Design review of the part built by this model. Coordinates are the model's own, in mm. Coordinates: 2 decimals unless noted, no trailing zeros. Write each loop counter-clockwise with the first axis right and the second up, starting at its lowest first coordinate (ties: lowest second). Pieces come first, ordered by that corner, then holes.
Q1. Take a section at B-B, the plane z = 11.5. Write out the cut boundary in (x, y), plus the area to 3 significant figures.
Q2. For L1, parallel to Y at x = 273.5, z = 12; L2, parallel to X at y = 145.5, z = 2.5; L3, parallel to X at y = 155, z = 15.5, list the stretches that pass through material, from the lowest coordinate up.
Q3. Take a section at A-A, the plane y = 76. Write out the cut boundary in (x, z), plus the area to 3 significant figures.
Q4. The part is to be moulded in two halves that separate along X. For faces 1 (the flat face through (804, 13, 3)), 2 (the flat face through (796, 11, 0)), say which applies: released by +X, released by -X, zero draft, split by the parting line, or undercut.
Q5. For pin 1 Ø12.5 at (x, z) = (1153.5, 11) entering from +Y; pin 2 Ø6.5 at (x, y) = (1587, 615.5) entering from +Z, all flat-tipped, find the tip position at first contact; note any pin that passes through.
Q6. Take a section at C-C, the plane x = 1246.5. Write out the cut boundary in (y, z), plus the area to 3 significant figures.
from build123d import *

# Parameters (mm, degrees)
F1_DEPTH = 1600
F3_DEPTH = 650
F5_DEPTH = 1600
F7_DEPTH = 650


with BuildPart() as f1:
    # F0 (on Right) → F1 (new body)
    with BuildSketch(Plane.YZ):
        Polygon((0, 25), (0, 0), (25, 0), (25, 3), (3, 3), (3, 25), align=None)
    extrude(amount=F1_DEPTH)

    # F2 (on Front) → F3 (join)
    with BuildSketch(Plane.XZ):
        Polygon((0, 25), (0, 0), (25, 0), (25, 3), (3, 3), (3, 25), align=None)
    extrude(amount=-F3_DEPTH)

    # F4 (on Right) → F5 (join)
    with BuildSketch(Plane.YZ):
        Polygon((600, 0), (600, 25), (597, 25), (597, 3), (575, 3), (575, 0), align=None)
    extrude(amount=F5_DEPTH)

    # F6 (on Front) → F7 (join)
    with BuildSketch(Plane.XZ):
        Polygon((1600, 0), (1600, 25), (1597, 25), (1597, 3), (1575, 3), (1575, 0), align=None)
    extrude(amount=-F7_DEPTH)


solid = f1.part
Responses:
1. outline: (0, 0) - (1600, 0) - (1600, 650) - (1597, 650) - (1597, 600) - (3, 600) - (3, 650) - (0, 650) - close; hole (3, 3) - (1597, 3) - (1597, 597) - (3, 597) - close
1. area: 13,500 mm2
2. L1: y = 0 to 3, 597 to 600
2. L2: x = 0 to 25, 1575 to 1600
2. L3: x = 0 to 3, 1597 to 1600
3. outline: (0, 0) - (25, 0) - (25, 3) - (3, 3) - (3, 25) - (0, 25) - close; (1575, 0) - (1600, 0) - (1600, 25) - (1597, 25) - (1597, 3) - (1575, 3) - close
3. area: 282 mm2
4. face 1: undercut
4. face 2: zero draft
5. pin 1: stops at y = 600
5. pin 2: stops at z = 3
6. outline: (0, 0) - (25, 0) - (25, 3) - (3, 3) - (3, 25) - (0, 25) - close; (575, 0) - (600, 0) - (600, 25) - (597, 25) - (597, 3) - (575, 3) - close
6. area: 282 mm2
